Check sheet for the modelled part. Datum: model origin and axes. Units: mm. A direction names the side the tool comes from. Give positions to 0.01 mm unless a question says otherwise; leave off trailing zeros. Order: outer loops, then holes, each group sorted by start corner. A loop starts at its lowest first (then second) coordinate and runs counter-clockwise, first axis right, second up.
```python
from build123d import *

# Parameters (mm, degrees)
BOSS_EXTRU_1_DEPTH = 10
ESQUISSE2_W        = 10
ESQUISSE2_H        = 45
BOSS_EXTRU_2_DEPTH = 10
CONG_1_R           = 20
BOSS_EXTRU_3_DEPTH = 10


with BuildPart() as part:
    # Esquisse1 → Boss.-Extru.1 (new body)
    with BuildSketch(Plane(origin=(0, 0, 0), x_dir=(1, 0, 0), z_dir=(0, 1, 0))):
        with BuildLine():
            Line((0, 0), (210, 0))
            Line((210, 0), (210, 40))
            ThreePointArc((210, 40), (202.5, 47.5), (195, 40))
            ThreePointArc((195, 40), (170, 15), (145, 40))
            ThreePointArc((145, 40), (137.5, 47.5), (130, 40))
            ThreePointArc((130, 40), (105, 15), (80, 40))
            ThreePointArc((80, 40), (72.5, 47.5), (65, 40))
            ThreePointArc((65, 40), (40, 15), (15, 40))
            ThreePointArc((15, 40), (7.5, 47.5), (0, 40))
            Line((0, 40), (0, 0))
        make_face()
    extrude(amount=BOSS_EXTRU_1_DEPTH)

    # Esquisse2 → Boss.-Extru.2 (add)
    with BuildSketch(Plane(origin=(0, 10, 0), x_dir=(1, 0, 0), z_dir=(0, 1, 0))):
        Polygon((60, -45), (50, -45), (45, -45), (45, -52), (65, -52), (65, -45), align=None)
        with Locations((55, -22.5)):
            Rectangle(ESQUISSE2_W, ESQUISSE2_H)
        with Locations((105, -22.5)):
            Rectangle(ESQUISSE2_W, ESQUISSE2_H)
        with Locations((155, -22.5)):
            Rectangle(ESQUISSE2_W, ESQUISSE2_H)
        Polygon((160, -45), (150, -45), (145, -45), (145, -52), (165, -52), (165, -45), align=None)
    extrude(amount=-BOSS_EXTRU_2_DEPTH)

    # Congé1
    cong_1_edges = [part.edges().sort_by_distance(p)[0] for p in [
        (210, 5, 0),
        (0, 5, 0),
    ]]
    fillet(cong_1_edges, radius=CONG_1_R)

    # Esquisse3 → Boss.-Extru.3 (add)
    with BuildSketch(Plane.ZY.offset(-100)):
        Polygon((3.209033432, 14.25), (4.755906928, 10), (6.283, 10), (7.829873496, 14.25), (9.492033432, 14.25), (11.038906928, 10), (12.566, 10), (14.112873496, 14.25), (15.775033432, 14.25), (17.321906928, 10), (18.849, 10), (20.395873496, 14.25), (22.058033432, 14.25), (23.604906928, 10), (25.132, 10), (26.678873496, 14.25), (28.341033432, 14.25), (29.887906928, 10), (31.415, 10), (32.961873496, 14.25), (34.624033432, 14.25), (36.170906928, 10), (37.698, 10), (39.244873496, 14.25), (40.907033432, 14.25), (42.453906928, 10), (43.981, 10), (45.527873496, 14.25), (47.190033432, 14.25), (48.736906928, 10), (50.264, 10), (51.810873496, 14.25), (53.473033432, 14.25), (55.019906928, 10), (56.547, 10), (58.093873496, 14.25), (59.756033432, 14.25), (61.302906928, 10), (62.83, 10), (64.376873496, 14.25), (66.039033432, 14.25), (67.585906928, 10), (69.113, 10), (70.659873496, 14.25), (72.322033432, 14.25), (73.868906928, 10), (75.396, 10), (76.942873496, 14.25), (78.605033432, 14.25), (80.151906928, 10), (81.679, 10), (83.225873496, 14.25), (84.888033432, 14.25), (86.434906928, 10), (87.962, 10), (89.508873496, 14.25), (91.171033432, 14.25), (92.717906928, 10), (94.245, 10), (95.791873496, 14.25), (97.454033432, 14.25), (99.000906928, 10), (100.528, 10), (102.074873496, 14.25), (103.737033432, 14.25), (105.283906928, 10), (106.811, 10), (108.357873496, 14.25), (110.020033432, 14.25), (111.566906928, 10), (113.094, 10), (114.640873496, 14.25), (116.303033432, 14.25), (117.849906928, 10), (119.377, 10), (120.923873496, 14.25), (122.586033432, 14.25), (124.132906928, 10), (125.66, 10), (125.66, 0), (0, 0), (0, 10), (1.546873496, 14.25), align=None)
    extrude(amount=-BOSS_EXTRU_3_DEPTH)


solid = part.part
```
(1) Material ranges on L1, parallel to X at y = 3.5, z = 46; L2, parallel to X at y = 5.75, z = 36; L3, parallel to X at y = 9, z = -18.5, recorded low to high.
Response values:
L1: x = 45 to 65, 100 to 110, 145 to 165
L2: x = 50 to 60, 100 to 110, 150 to 160
L3: x = 0.06 to 27.24, 52.76 to 92.24, 117.76 to 157.24, 182.76 to 209.94
(2) Set-up check for faces 4 (the face through (45, 5, 48)), 5 (the face through (63, 5, 45)), 6 (the face through (104.93, 12.095, 19.612)), 7 (the face through (163, 5, 45)), 8 (the face through (105, 5, 125.66)): record each of +Z, -Z, +X, -X, +Y, -Y from which the full face is reachable in a straight line by a thin tool's end or side.
Response values:
face 4: +Z, -X, +Y, -Y
face 5: +Y, -Y
face 6: +X, -X, +Y
face 7: +X, +Y, -Y
face 8: +Z, +X, -X, +Y, -Y
(3) Gauge pin test, flat ends, axial feed: pin 1 Ø2 at (y, z) = (7, 101.5) entering from -X; pin 2 Ø5 at (y, z) = (4.5, 11.5) entering from +X; pin 3 Ø0.8 at (x, z) = (103, 62) entering from +Y; pin 4 Ø1.5 at (x, y) = (67.5, 11) entering from +Z. Record the tip position at first contact, or that the pin passes through.
Response values:
pin 1: stops at x = 100
pin 2: stops at x = 160
pin 3: stops at y = 10
pin 4: passes through
(4) Release check for a two-part mould opening along X. For faces 1 (the face through (50, 5, 23)), 2 (the face through (80, 5, 0)), 3 (the face through (104.93, 12.15, 35.39)) record: released by +X, released by -X, zero draft, split by the parting line, or undercut.
Response values:
face 1: released by -X
face 2: undercut
face 3: zero draft
(5) Cross-section at B-B on x = 40. Enter the section's corners in (y, z).
Response values:
outline: (0, -15) - (10, -15) - (10, 0) - (0, 0) - close
(6) Cross-section at C-C on x = 137.5. Enter the section's corners in (y, z), then the cut area to 3 significant figures.
Response values:
outline: (0, -47.5) - (10, -47.5) - (10, 0) - (0, 0) - close
area: 475 mm2
